from build123d import *

# Parameters (mm, degrees)
SKETCH_1_R      = 117.5
SKETCH_1_R_2    = 85
SKETCH_1_R_3    = 4.5
EXTRUDE_1_DEPTH = 4
SCALE_1_SCALE   = 0.2


with BuildPart() as part:
    # 草图1 → 凸台-拉伸1 (new body)
    with BuildSketch(Plane.XY):
        Circle(SKETCH_1_R)
        Circle(SKETCH_1_R_2, mode=Mode.SUBTRACT)
        with Locations((0, 100)):
            Circle(SKETCH_1_R_3, mode=Mode.SUBTRACT)
        with Locations((86.602540378, 50)):
            Circle(SKETCH_1_R_3, mode=Mode.SUBTRACT)
        with Locations((86.602540378, -50)):
            Circle(SKETCH_1_R_3, mode=Mode.SUBTRACT)
        with Locations((0, -100)):
            Circle(SKETCH_1_R_3, mode=Mode.SUBTRACT)
        with Locations((-86.602540378, -50)):
            Circle(SKETCH_1_R_3, mode=Mode.SUBTRACT)
        with Locations((-86.602540378, 50)):
            Circle(SKETCH_1_R_3, mode=Mode.SUBTRACT)
    extrude(amount=EXTRUDE_1_DEPTH)


with BuildPart() as part_1:
    # 缩放比例1: scaled about (0, 0, 2)
    add(part.part.scale(SCALE_1_SCALE).moved(Location((0, 0, 1.6))))


solid = part_1.part
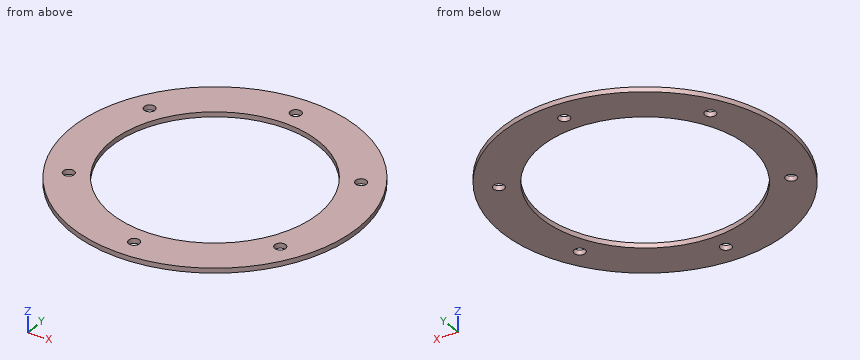
Check sheet for the modelled part. Datum: model origin and axes. Units: mm. Round coordinates to 2 decimals unless told otherwise and drop trailing zeros. Order: outer loops, then holes, each group sorted by start corner. A loop starts at its lowest first (then second) coordinate and runs counter-clockwise, first axis right, second up.
Q1. Cross-section at C-C, the plane z = 2. Enter the section's corners in (x, y).
Filled sheet:
outline: circle Ø47 at (0, 0); hole circle Ø1.8 at (-17.32, -10); hole circle Ø1.8 at (-17.32, 10); hole circle Ø34 at (0, 0); hole circle Ø1.8 at (0, -20); hole circle Ø1.8 at (0, 20); hole circle Ø1.8 at (17.32, -10); hole circle Ø1.8 at (17.32, 10)
Q2. Cross-section at A-A, the plane y = 0. Enter the section's corners in (x, z), plus the area to 3 significant figures.
Filled sheet:
outline: (-23.5, 1.6) - (-17, 1.6) - (-17, 2.4) - (-23.5, 2.4) - close; (17, 1.6) - (23.5, 1.6) - (23.5, 2.4) - (17, 2.4) - close
area: 10.4 mm2
Q3. Cross-section at D-D, the plane x = 6.5. Enter the section's corners in (y, z).
Filled sheet:
outline: (-22.58, 1.6) - (-15.71, 1.6) - (-15.71, 2.4) - (-22.58, 2.4) - close; (15.71, 1.6) - (22.58, 1.6) - (22.58, 2.4) - (15.71, 2.4) - close
Q4. Depth check by flat-ended pin: P1, Ø1.4, axis at x = -17.32, y = 10, coming from the +Z side. Enter the tip coordinate at first touch or a pass-through.
Filled sheet:
P1: passes through
Q5. Scan lines: L1, parallel to Y at x = 0, z = 2.2; L2, parallel to X at y = 10, z = 2.25; L3, parallel to X at y = 20, z = 1.95. Record each from-to range of solid material in increasing order.
Filled sheet:
L1: y = -23.5 to -20.9, -19.1 to -17, 17 to 19.1, 20.9 to 23.5
L2: x = -21.27 to -18.22, -16.42 to -13.75, 13.75 to 16.42, 18.22 to 21.27
L3: x = -12.34 to -0.9, 0.9 to 12.34
Q6. Cross-section at B-B, the plane x = 0. Enter the section's corners in (y, z).
Filled sheet:
outline: (-23.5, 1.6) - (-20.9, 1.6) - (-20.9, 2.4) - (-23.5, 2.4) - close; (-19.1, 1.6) - (-17, 1.6) - (-17, 2.4) - (-19.1, 2.4) - close; (17, 1.6) - (19.1, 1.6) - (19.1, 2.4) - (17, 2.4) - close; (20.9, 1.6) - (23.5, 1.6) - (23.5, 2.4) - (20.9, 2.4) - close
